For this review, take the finished solid that the model builds, in its own axes (mm). Round coordinates to 2 decimals unless told otherwise and drop trailing zeros. Loops run counter-clockwise (first coordinate to the right, second up) from the corner with the lowest first, then second, coordinate; pieces in that order, holes last.
1. Consider section B-B on z = -0.4. State how many separate pieces and enclosed holes the cut face has, then the cut area to 3 significant figures.
2. Consider section A-A on y = -34.5. State the section outline as (x, z) points (3 decimals).
3. Clearance check with a flat-ended pin moving along its axis: pin 1 Ø2 at (x, y) = (-50, 50) entering from +Z. State where the tip first meets the part, or that it passes through.
4. To check wall thickness, follow line 1 along X through (y, z) = (-8.5, -0.5) (3 decimals); line 2 along Y through (x, z) = (50, -0.8) (3 decimals); line 3 along Y through (x, z) = (11.5, -0.15) (3 decimals). State the ranges of each line that lie inside material, in increasing order.
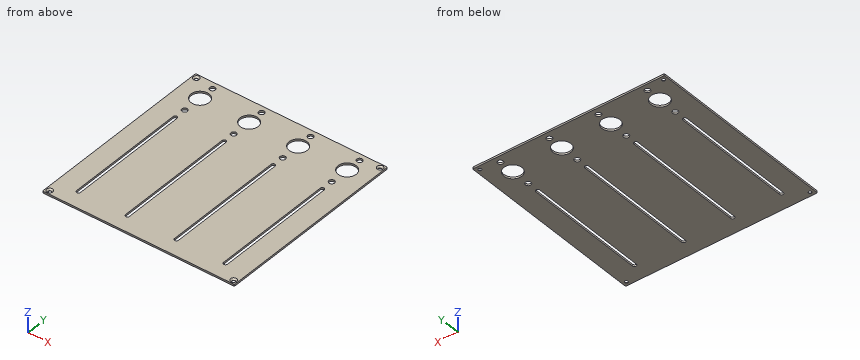
from build123d import *

# Parameters (mm, degrees)
PAD_DEPTH        = 1
POCKET_DEPTH     = 0.001
HOLE_D           = 1.75
HOLE_CSINK_D     = 3.3
HOLE_CSINK_ANGLE = 90
SKETCH020_R      = 4.9
HOLE012_DEPTH    = 1.001
POCKET006_DEPTH  = 1.001
SKETCH022_R      = 1.5
HOLE013_DEPTH    = 1.001


with BuildPart() as part:
    # Sketch → Pad (new body)
    with BuildSketch(Plane.XY):
        with BuildLine():
            Line((-51.8, 52.175), (51.8, 52.175))
            ThreePointArc((52.175, 51.8), (52.065165, 52.065165), (51.8, 52.175))
            Line((52.175, 51.8), (52.175, -51.8))
            ThreePointArc((51.8, -52.175), (52.065165, -52.065165), (52.175, -51.8))
            Line((51.8, -52.175), (-51.8, -52.175))
            ThreePointArc((-52.175, -51.8), (-52.065165, -52.065165), (-51.8, -52.175))
            Line((-52.175, -51.8), (-52.175, 51.8))
            ThreePointArc((-51.8, 52.175), (-52.065165, 52.065165), (-52.175, 51.8))
        make_face()
    extrude(amount=-PAD_DEPTH)

    # Sketch002 → Pocket (cut, through all)
    with BuildSketch(Plane.XY.offset(-4.8)):
        with BuildLine():
            Line((-45, 50.175), (45, 50.175))
            ThreePointArc((45, 50.175), (45.353553, 50.321447), (45.5, 50.675))
            ThreePointArc((45.5, 50.675), (45.353553, 51.028553), (45, 51.175))
            Line((-45, 51.175), (45, 51.175))
            ThreePointArc((-45, 51.175), (-45.353553, 51.028553), (-45.5, 50.675))
            ThreePointArc((-45.5, 50.675), (-45.353553, 50.321447), (-45, 50.175))
        make_face()
        with BuildLine():
            Line((-45, -51.175), (45, -51.175))
            ThreePointArc((45, -51.175), (45.353553, -51.028553), (45.5, -50.675))
            ThreePointArc((45.5, -50.675), (45.353553, -50.321447), (45, -50.175))
            Line((-45, -50.175), (45, -50.175))
            ThreePointArc((-45, -50.175), (-45.353553, -50.321447), (-45.5, -50.675))
            ThreePointArc((-45.5, -50.675), (-45.353553, -51.028553), (-45, -51.175))
        make_face()
        with BuildLine():
            Line((51.175, -45), (51.175, 45))
            ThreePointArc((51.175, 45), (51.028553, 45.353553), (50.675, 45.5))
            ThreePointArc((50.675, 45.5), (50.321447, 45.353553), (50.175, 45))
            Line((50.175, -45), (50.175, 45))
            ThreePointArc((50.175, -45), (50.321447, -45.353553), (50.675, -45.5))
            ThreePointArc((50.675, -45.5), (51.028553, -45.353553), (51.175, -45))
        make_face()
        with BuildLine():
            Line((-50.175, -45), (-50.175, 45))
            ThreePointArc((-50.175, 45), (-50.321447, 45.353553), (-50.675, 45.5))
            ThreePointArc((-50.675, 45.5), (-51.028553, 45.353553), (-51.175, 45))
            Line((-51.175, -45), (-51.175, 45))
            ThreePointArc((-51.175, -45), (-51.028553, -45.353553), (-50.675, -45.5))
            ThreePointArc((-50.675, -45.5), (-50.321447, -45.353553), (-50.175, -45))
        make_face()
    extrude(amount=-POCKET_DEPTH, mode=Mode.SUBTRACT)

    # Hole (through all)
    with Locations(Plane.XY):
        with Locations((-50, 50), (50, 50), (50, -50), (-50, -50)):
            CounterSinkHole(HOLE_D / 2, HOLE_CSINK_D / 2, counter_sink_angle=HOLE_CSINK_ANGLE)

    # Sketch020 → Hole012 (cut, through all)
    with BuildSketch(Plane.XY):
        with Locations((-40.005, 40.005)):
            Circle(SKETCH020_R)
        with Locations((-13.335, 40.005)):
            Circle(SKETCH020_R)
        with Locations((13.335, 40.005)):
            Circle(SKETCH020_R)
        with Locations((40.005, 40.005)):
            Circle(SKETCH020_R)
    extrude(amount=-HOLE012_DEPTH, mode=Mode.SUBTRACT)

    # Sketch021 → Pocket006 (cut, through all)
    with BuildSketch(Plane.XY):
        with BuildLine():
            ThreePointArc((-38.955, 23), (-40.005, 24.05), (-41.055, 23))
            Line((-41.055, 23), (-41.055, -43))
            ThreePointArc((-41.055, -43), (-40.005, -44.05), (-38.955, -43))
            Line((-38.955, 23), (-38.955, -43))
        make_face()
        with BuildLine():
            ThreePointArc((-12.285, 23), (-13.335, 24.05), (-14.385, 23))
            Line((-14.385, 23), (-14.385, -43))
            ThreePointArc((-14.385, -43), (-13.335, -44.05), (-12.285, -43))
            Line((-12.285, 23), (-12.285, -43))
        make_face()
        with BuildLine():
            ThreePointArc((14.385, 23), (13.335, 24.05), (12.285, 23))
            Line((12.285, 23), (12.285, -43))
            ThreePointArc((12.285, -43), (13.335, -44.05), (14.385, -43))
            Line((14.385, 23), (14.385, -43))
        make_face()
        with BuildLine():
            ThreePointArc((41.055, 23), (40.005, 24.05), (38.955, 23))
            Line((38.955, 23), (38.955, -43))
            ThreePointArc((38.955, -43), (40.005, -44.05), (41.055, -43))
            Line((41.055, 23), (41.055, -43))
        make_face()
    extrude(amount=-POCKET006_DEPTH, mode=Mode.SUBTRACT)

    # Sketch022 → Hole013 (cut, through all)
    with BuildSketch(Plane.XY):
        with Locations((-40.005, 48.505)):
            Circle(SKETCH022_R)
        with Locations((-13.335, 48.505)):
            Circle(SKETCH022_R)
        with Locations((13.335, 48.505)):
            Circle(SKETCH022_R)
        with Locations((40.005, 48.505)):
            Circle(SKETCH022_R)
        with Locations((-40.005, 29.5)):
            Circle(SKETCH022_R)
        with Locations((-13.335, 29.5)):
            Circle(SKETCH022_R)
        with Locations((13.335, 29.5)):
            Circle(SKETCH022_R)
        with Locations((40.005, 29.5)):
            Circle(SKETCH022_R)
    extrude(amount=-HOLE013_DEPTH, mode=Mode.SUBTRACT)


solid = part.part
Resolved:
1. separate pieces: 1
1. enclosed holes: 20
1. area: 9,940 mm2
2. outline: (-52.175, -1) - (-41.055, -1) - (-41.055, 0) - (-52.175, 0) - close; (-38.955, -1) - (-14.385, -1) - (-14.385, 0) - (-38.955, 0) - close; (-12.285, -1) - (12.285, -1) - (12.285, 0) - (-12.285, 0) - close; (14.385, -1) - (38.955, -1) - (38.955, 0) - (14.385, 0) - close; (41.055, -1) - (52.175, -1) - (52.175, 0) - (41.055, 0) - close
3. pin 1: stops at z = -0.65
4. line 1: x = -52.175 to -41.055, -38.955 to -14.385, -12.285 to 12.285, 14.385 to 38.955, 41.055 to 52.175
4. line 2: y = -52.175 to -50.875, -49.125 to 49.125, 50.875 to 52.175
4. line 3: y = -52.175 to 35.462, 44.548 to 52.175
